from build123d import *

# Parameters (mm, degrees)
F0_W     = 40
F0_H     = 30
F1_DEPTH = 15
F0_W_2   = 10
F2_DEPTH = 50
F3_W     = 10
F3_H     = 10
F4_DEPTH = 10
F5_R     = 2


with BuildPart() as f1:
    # F0 (on Top) → F1 (new body)
    with BuildSketch(Plane.XY):
        with Locations((5.999135, 2.211004)):
            Rectangle(F0_W, F0_H)
    extrude(amount=F1_DEPTH)

    # F0 (on Top) → F2 (join)
    with BuildSketch(Plane.XY):
        with Locations((-19.000865, 2.211004)):
            Rectangle(F0_W_2, F0_H)
    extrude(amount=F2_DEPTH)

    # F3 (on face) → F4 (cut)
    with BuildSketch(Plane.XY):
        with Locations((0.999135, 3.211004)):
            Rectangle(F3_W, F3_H)
    extrude(amount=F4_DEPTH, mode=Mode.SUBTRACT)

    # F5
    f5_edges = [f1.edges().sort_by_distance(p)[0] for p in [
        (-19.000865, -12.788996, 50),
        (-14.000865, 2.211004, 50),
        (-24.000865, 2.211004, 50),
        (-19.000865, 17.211004, 50),
        (5.999135, -12.788996, 15),
        (25.999135, 2.211004, 15),
        (5.999135, 17.211004, 15),
        (25.999135, 17.211004, 7.5),
        (25.999135, -12.788996, 7.5),
        (-24.000865, 17.211004, 25),
        (-24.000865, -12.788996, 25),
    ]]
    fillet(f5_edges, radius=F5_R)


solid = f1.part
Could you check a few things on this model? Use its own coordinates, in mm. A direction names the side the tool comes from. Coordinates: 2 decimals unless noted, no trailing zeros. Loops run counter-clockwise (first coordinate to the right, second up) from the corner with the lowest first, then second, coordinate; pieces in that order, holes last. Notation, with made-up numbers: (-15, -8) -> (-11, -8) arc R13 cw to (-11, 5) -> close; hole circle Ø7 at (-28, 14). An arc over 180 degrees is marked (long way). Answer in a Markdown table with one row per item.
(1) If I drill on probe 1 along Z at (x, y) = (4, 12.25); probe 2 along X at (y, z) = (7.5, 25); probe 3 along Z at (x, y) = (2.5, 6.75), over which ranges is the centre line in solid material (lowest first)?
Results found:
| item | result |
|---|---|
| probe 1 | z = 0 to 15 |
| probe 2 | x = -24 to -14 |
| probe 3 | z = 10 to 15 |
(2) Imagine slicing it at C-C (x = 2). List the corners of the cut face in (y, z) for me.
Results found:
| item | result |
|---|---|
| outline | (-12.79, 0) -> (-1.79, 0) -> (-1.79, 10) -> (8.21, 10) -> (8.21, 0) -> (17.21, 0) -> (17.21, 13) arc R2 ccw to (15.21, 15) -> (-10.79, 15) arc R2 ccw to (-12.79, 13) -> close |
(3) Imagine slicing it at B-B (y = -9). List the corners of the cut face in (x, z) for me, plus the area to 3 significant figures.
Results found:
| item | result |
|---|---|
| outline | (-24, 0) -> (26, 0) -> (26, 13) arc R2 ccw to (24, 15) -> (-14, 15) -> (-14, 48) arc R2 ccw to (-16, 50) -> (-22, 50) arc R2 ccw to (-24, 48) -> close |
| area | 1,100 mm^2 |
(4) Imagine slicing it at A-A (z = 4.5). List the corners of the cut face in (x, y) for me.
Results found:
| item | result |
|---|---|
| outline | (-24, -10.79) arc R2 ccw to (-22, -12.79) -> (24, -12.79) arc R2 ccw to (26, -10.79) -> (26, 15.21) arc R2 ccw to (24, 17.21) -> (-22, 17.21) arc R2 ccw to (-24, 15.21) -> close; hole (-4, -1.79) -> (6, -1.79) -> (6, 8.21) -> (-4, 8.21) -> close |
(5) Will these pins go through, and if not, where does the flat tip stop? pin 1 Ø5 at (y, z) = (-6.5, 37) entering from +X; pin 2 Ø2 at (x, y) = (-12, 4) entering from +Z.
Results found:
| item | result |
|---|---|
| pin 1 | stops at x = -14 |
| pin 2 | stops at z = 15 |
(6) Imagine slicing it at D-D (z = 28.5). List the corners of the cut face in (x, y) for me.
Results found:
| item | result |
|---|---|
| outline | (-24, -10.79) arc R2 ccw to (-22, -12.79) -> (-14, -12.79) -> (-14, 17.21) -> (-22, 17.21) arc R2 ccw to (-24, 15.21) -> close |
(7) For faces 1 (the face through (5.999, 3, 5)), 2 (the face through (5, 2, 15)), 3 (the face through (5.27, -12.22, 14.4)), 4 (the face through (-17.94, -12.22, 49.4)), 5 (the face through (-5, 2, 0)), which set-ups out of +Z, -Z, +X, -X, +Y, -Y let a thin tool reach every point of the face, with its end or its side?
Results found:
| item | result |
|---|---|
| face 1 | -Z |
| face 2 | +Z, +X, +Y, -Y |
| face 3 | +Z, +X, -Y |
| face 4 | +Z, +X, -X, -Y |
| face 5 | -Z, +X, -X, +Y, -Y |
(8) Thinking about a two-plate mould opening in Y: for faces 6 (the face through (1, 8.211, 5)), 7 (the face through (-4, -12.789, 8)), 8 (the face through (-23.43, 16.61, 24.34)), 9 (the face through (25.999, 2, 6)), which applies, released by +Y, released by -Y, zero draft, split by the parting line, or undercut?
Results found:
| item | result |
|---|---|
| face 6 | undercut |
| face 7 | released by -Y |
| face 8 | released by +Y |
| face 9 | zero draft |
